from build123d import *

# Parameters (mm, degrees)
SKETCH_2_W          = 100
SKETCH_2_H          = 100
EXTRUDE_1_DEPTH     = 10
FILLET_1_R          = 10
SHELL_START         = 5
SHELL_1_OUTLINE_R   = 25
SHELL_1_DEPTH       = 1040
SHELL_START_2       = 1045
SHELL_1_2_OUTLINE_R = 20
SHELL_1_2_DEPTH     = 205


# Read off the part's stored shape, not the designer's step: 抽壳1
with BuildPart() as part:
    # 草图1 → 旋转1 (revolve)
    with BuildSketch(Plane.XY, mode=Mode.PRIVATE) as revolve_1_sk:
        Polygon((0, 0), (30, 0), (30, 1050), (25, 1050), (25, 1250), (0, 1250), align=None)
    revolve(revolve_1_sk.sketch.rotate(Axis((0, 1250, 0), (0, -1, 0)), 180), axis=Axis((0, 1250, 0), (0, -1, 0)))

    # 草图2 → 凸台-拉伸1 (add)
    with BuildSketch(Plane.XZ):
        Rectangle(SKETCH_2_W, SKETCH_2_H)
    extrude(amount=-EXTRUDE_1_DEPTH)

    # 圆角1
    fillet_1_edges = [part.edges().sort_by_distance(p)[0] for p in [
        (50, 5, 50),
        (50, 5, -50),
        (-50, 5, -50),
        (-50, 5, 50),
    ]]
    fillet(fillet_1_edges, radius=FILLET_1_R)

    # 抽壳1 outline → 抽壳1 (cut)
    with BuildSketch(Plane(origin=(0, 0, 0), x_dir=(1, 0, 0), z_dir=(0, 1, 0)).offset(SHELL_START)):
        Circle(SHELL_1_OUTLINE_R)
    extrude(amount=SHELL_1_DEPTH, mode=Mode.SUBTRACT)

    # Shell 1 2 outline → Shell 1 2 (cut)
    with BuildSketch(Plane(origin=(0, 0, 0), x_dir=(1, 0, 0), z_dir=(0, 1, 0)).offset(SHELL_START_2)):
        Circle(SHELL_1_2_OUTLINE_R)
    extrude(amount=SHELL_1_2_DEPTH, mode=Mode.SUBTRACT)


solid = part.part
The model under review builds one solid part; all positions refer to its coordinate system, in mm. A direction names the side the tool comes from. Round coordinates to 2 decimals unless told otherwise and drop trailing zeros. Loops run counter-clockwise (first coordinate to the right, second up) from the corner with the lowest first, then second, coordinate; pieces in that order, holes last. Notation, with made-up numbers: (8, -11.75) -> (27, -11.75) arc R26 cw to (27, 2.25) -> close; hole circle Ø2 at (27.5, 19.5). An arc over 180 degrees is marked (long way). Write item = value, one per line. Start each with the question number.
Item 1: Take a section at A-A on z = 0. Give the boundary of the cut face in (x, y), plus the area to 3 significant figures.
Item 2: To check wall thickness, follow L1, parallel to Z at x = 0, y = 1195; L2, parallel to Y at x = 22, z = -1; L3, parallel to Y at x = -32.5, z = -43. State the ranges of each line that lie inside material, in increasing order.
Item 3: Take a section at C-C on y = 854.5. Give the boundary of the cut face in (x, z).
Item 4: Insertion check: pin 1 (5 mm diameter, centred on x = 3.5, y = 601.5, fed in from -Z); pin 2 (1.5 mm diameter, centred on x = -9.5, z = -28, fed in from -Y); pin 3 (3 mm diameter, centred on y = 694, z = 12, fed in from -X); pin 4 (3 mm diameter, centred on x = 2.5, z = -12.5, fed in from +Y). Each pin has a flat end and moves straight along its axis. Give the tip position at first contact, or say it passes through.
Item 5: For faces 4 (the flat face through (11, 1250, -17)), 5 (the flat face through (0, 5, 0)), 6 (the cylindrical face through (-16.128, 537.28, -25.296)), list the 3-axis set-ups (+Z, -Z, +X, -X, +Y, -Y) from which the entire face can be reached by the end or side of a thin tool; tool diameter is ignored.
Item 6: Mouldability with a two-part tool opening along Y and no side actions: class faces 1 (the flat face through (-1, 0, 1)), 2 (the cylindrical face through (23.846, 517.72, -7.509)), 3 (the flat face through (7, 1050, -25)) as released by +Y, released by -Y, zero draft, split by the parting line, or undercut.
Item 7: Take a section at B-B on x = 0. Give the boundary of the cut face in (y, z).
Result:
q1.outline = (-50, 0) -> (50, 0) -> (50, 10) -> (30, 10) -> (30, 1050) -> (25, 1050) -> (25, 1250) -> (20, 1250) -> (20, 1045) -> (25, 1045) -> (25, 5) -> (-25, 5) -> (-25, 1045) -> (-20, 1045) -> (-20, 1250) -> (-25, 1250) -> (-25, 1050) -> (-30, 1050) -> (-30, 10) -> (-50, 10) -> close
q1.area = 13,200 mm²
q2.L1 = -25 to -20, 20 to 25
q2.L2 = 0 to 5, 1045 to 1250
q2.L3 = 0 to 10
q3.outline = circle Ø60 at (0, 0); hole circle Ø50 at (0, 0)
q4.pin_1 = -29.98
q4.pin_2 = 0
q4.pin_3 = -28.1
q4.pin_4 = 5
q5.face_4 = +Z, -Z, +X, -X, +Y
q5.face_5 = none
q5.face_6 = +Y
q6.face_1 = released by -Y
q6.face_2 = undercut
q6.face_3 = released by +Y
q7.outline = (0, -50) -> (10, -50) -> (10, -30) -> (1050, -30) -> (1050, -25) -> (1250, -25) -> (1250, -20) -> (1045, -20) -> (1045, -25) -> (5, -25) -> (5, 25) -> (1045, 25) -> (1045, 20) -> (1250, 20) -> (1250, 25) -> (1050, 25) -> (1050, 30) -> (10, 30) -> (10, 50) -> (0, 50) -> close
